Geometry check sheet. Reference: the model listing, model coordinates, mm. A direction names the side the tool comes from. Give positions to 0.01 mm unless a question says otherwise; leave off trailing zeros. Loops run counter-clockwise (first coordinate to the right, second up) from the corner with the lowest first, then second, coordinate; pieces in that order, holes last. Notation, with made-up numbers: (63, 43.5) - (119, 43.5) arc R9 ccw to (119, 58.5) - close; hole circle Ø6 at (-20, -31). An arc over 180 degrees is marked (long way). Use a Markdown table: item, result. Add a question column.
1. Depth check by flat-ended pin: P1, Ø1, axis at y = -4, z = 0.5, coming from the +X side; P2, Ø1.2, axis at x = -37, z = 2, coming from the +Y side; P3, Ø1.2, axis at y = -24.5, z = 1.5, coming from the -X side. Enter the tip coordinate at first touch or a pass-through.
2. Material ranges on L1, parallel to X at y = -24.5, z = 0.7; L2, parallel to Y at x = -10.5, z = 1; L3, parallel to X at y = -20.5, z = 2.45, recorded low to high.
3. Cross-section at B-B on y = 1. Enter the section's corners in (x, z), and give its area (3 significant figures).
4. Draft check along Y on faces 1 (the flat face through (0, 22.5, 2)), 2 (the flat face through (0, -22.5, 2)), 3 (the flat face through (32.5, 24, 2)), 4 (the flat face through (45, 7.5, 2)). Enter one of: pulls with the +Y half, pulls with the -Y half, needs draft (parallel to the pull), parting line crosses it, or undercut.
5. Set-up check for faces 5 (the flat face through (-38, 22.5, 2)), 6 (the flat face through (44, 17.8, 2)), 7 (the flat face through (38, -22.5, 2)), 8 (the flat face through (-32.8, -27, 2)), 9 (the flat face through (22.2, -27, 2)): record each of +Z, -Z, +X, -X, +Y, -Y from which the full face is reachable in a straight line by a thin tool's end or side.
6. Cross-section at C-C on x = -8. Enter the section's corners in (y, z).
7. Cross-section at A-A on y = -26. Enter the section's corners in (x, z).
Autodesk Inventor part; units mm, degrees
ref_plane "Work Plane1" through (0, -7.2, 0) normal (1, 0, 0) x (0, 0, -1)
ref_plane "YZ Plane" through (0, 0, 0) normal (1, 0, 0) x (0, 1, 0)
ref_plane "XZ Plane" through (0, 0, 0) normal (0, 1, 0) x (-1, 0, 0)
sketch "Sketch1" plane through (0, 0, 0) normal (0, 0, 1) x (1, 0, 0)
  line L0 (42.5, -22.5) -> (-42.5, -22.5)
  line L1 (-42.5, -22.5) -> (-42.5, 22.5)
  line L2 (-42.5, 22.5) -> (42.5, 22.5)
  line L3 (42.5, 22.5) -> (42.5, -22.5)
  line L4 (42.5, -22.5) -> (-42.5, 22.5) construction
  line L5 (-42.5, -22.5) -> (42.5, 22.5) construction
  point P0 (0, 0)
  dimension "d0" = 85
  dimension "d1" = 45
extrude "Extrusion1" add sketch "Sketch1" along normal blind 4
sketch "Sketch2" plane through (0, 0, 4) normal (0, 0, 1) x (1, 0, 0)
  line L0 (-42.5, -22.5) -> (42.5, -22.5)
  line L1 (42.5, -22.5) -> (42.5, 22.5)
  line L2 (42.5, 22.5) -> (-42.5, 22.5)
  line L3 (-42.5, 22.5) -> (-42.5, -22.5)
  line L4 (42.5, -22.5) -> (42.5, 22.5)
  line L5 (42.5, 17.8) -> (46.5, 17.8)
  line L6 (46.5, 17.8) -> (46.5, 7.5)
  line L7 (46.5, 7.5) -> (42.5, 7.5)
  line L8 (42.5, 7.5) -> (42.5, 17.8)
  line L9 (42.5, -7.2) -> (46.5, -7.2)
  line L10 (46.5, -7.2) -> (46.5, -17.5)
  line L11 (46.5, -17.5) -> (42.5, -17.5)
  line L12 (42.5, -17.5) -> (42.5, -7.2)
  point P0 (0, 0)
  dimension "d4" = 4
  dimension "d5" = 10.3
  dimension "d6" = 4
  dimension "d7" = 10.3
extrude "Extrusion2" add sketch "Sketch2" against normal blind 4 contours L1 L9 L10 L11 | L5 L6 L7 L1
ref_plane "Work Plane1" through (0, -7.2, 0) normal (1, 0, 0) x (0, 0, -1)
mirror "Mirror1" about plane through (0, -7.2, 0) normal (1, 0, 0) of "Extrusion2"
sketch "Sketch3" plane through (0, 0, 4) normal (0, 0, 1) x (1, 0, 0)
  line L0 (-42.5, -22.5) -> (42.5, -22.5)
  line L1 (-32.8, -22.5) -> (-22.5, -22.5)
  line L2 (-22.5, -22.5) -> (-22.5, -30.5)
  line L3 (-22.5, -30.5) -> (-32.8, -30.5)
  line L4 (-32.8, -30.5) -> (-32.8, -22.5)
  line L5 (22.2, -22.5) -> (32.5, -22.5)
  line L6 (32.5, -22.5) -> (32.5, -30.5)
  line L7 (32.5, -30.5) -> (22.2, -30.5)
  line L8 (22.2, -30.5) -> (22.2, -22.5)
  line L9 (-42.5, -17.5) -> (-42.5, -22.5)
  line L10 (42.5, -22.5) -> (42.5, -17.5)
  point P0 (0, 0)
  dimension "d12" = 10.3
  dimension "d13" = 8
  dimension "d14" = 10.3
  dimension "d15" = 8
extrude "Extrusion3" add sketch "Sketch3" against normal blind 4
sketch "Sketch5" plane through (0, 0, 4) normal (0, 0, 1) x (1, 0, 0)
  line L0 (42.5, 22.5) -> (-42.5, 22.5)
  line L1 (-32.8, 22.5) -> (-22.5, 22.5)
  line L2 (-22.5, 22.5) -> (-22.5, 26.5)
  line L3 (-22.5, 26.5) -> (-32.8, 26.5)
  line L4 (-32.8, 26.5) -> (-32.8, 22.5)
  line L5 (22.2, 22.5) -> (32.5, 22.5)
  line L6 (32.5, 22.5) -> (32.5, 26.5)
  line L7 (32.5, 26.5) -> (22.2, 26.5)
  line L8 (22.2, 26.5) -> (22.2, 22.5)
  line L9 (-42.5, 22.5) -> (-42.5, 17.8)
  line L10 (42.5, 17.8) -> (42.5, 22.5)
  point P0 (0, 0)
  dimension "d20" = 10.3
  dimension "d21" = 4
  dimension "d22" = 10.3
  dimension "d23" = 4
extrude "Extrusion4" add sketch "Sketch5" against normal blind 4
equation "\"d5\" = d"
equation "\"d7\" = d"
equation "\"d12\" = d"
equation "\"d14\" = d"
equation "\"d20\" = d"
equation "\"d22\" = d"
equation "\"d\" = 10.3"
properties part number "FUENTE 2-02"
Values found:
| question | item | result |
|---|---|---|
| 1 | P1 | stops at x = 42.5 |
| 1 | P2 | stops at y = 22.5 |
| 1 | P3 | stops at x = -32.8 |
| 2 | L1 | x = -32.8 to -22.5, 22.2 to 32.5 |
| 2 | L2 | y = -22.5 to 22.5 |
| 2 | L3 | x = -42.5 to 42.5 |
| 3 | outline | (-42.5, 0) - (42.5, 0) - (42.5, 4) - (-42.5, 4) - close |
| 3 | area | 340 mm2 |
| 4 | face 1 | pulls with the +Y half |
| 4 | face 2 | pulls with the -Y half |
| 4 | face 3 | needs draft |
| 4 | face 4 | undercut |
| 5 | face 5 | +Z, -Z, -X, +Y |
| 5 | face 6 | +Z, -Z, +X, +Y |
| 5 | face 7 | +Z, -Z, +X, -Y |
| 5 | face 8 | +Z, -Z, -X, -Y |
| 5 | face 9 | +Z, -Z, -Y |
| 6 | outline | (-22.5, 0) - (22.5, 0) - (22.5, 4) - (-22.5, 4) - close |
| 7 | outline | (-32.8, 0) - (-22.5, 0) - (-22.5, 4) - (-32.8, 4) - close; (22.2, 0) - (32.5, 0) - (32.5, 4) - (22.2, 4) - close |
